Build history of the part. All positions in model axes, mm. A direction names the side the tool comes from. Coordinates: 2 decimals unless noted, no trailing zeros. Write each loop counter-clockwise with the first axis right and the second up, starting at its lowest first coordinate (ties: lowest second). Pieces come first, ordered by that corner, then holes. Notation, with made-up numbers: (-13, -24.75) -> (-2, -24.75) arc R19 cw to (-2, -17.75) -> close; hole circle Ø7 at (87.25, 64.25). An arc over 180 degrees is marked (long way). Write each question's results on one line, items separated by ' | '. Start each with the question number.
Q1. Two-plate mould, pull along Y, no slides. Class faces 1 (the face through (13, 17, 3)), 2 (the face through (10, 24, 6)), 3 (the face through (16.403, 18, 1)), 4 (the face through (11.403, 8, 1)): released by +Y, released by -Y, zero draft, split by the parting line, or undercut.
Q2. Drill centre lines: line 1 (X direction, y = 9.5, z = -2.25); line 2 (Y direction, x = 12, z = 4.5); line 3 (Y direction, x = 4, z = 5.5). Where is each one in solid material? Low to high.
Q3. Tool access for faces 5 (the face through (-11.597, 22, 1)), 6 (the face through (13, 19.5, 3)), 7 (the face through (11.4, 26.22, 1.47)): list every direction of +Z, -Z, +X, -X, +Y, -Y with a clear straight run to the whole face (end or side of a thin tool).
Q4. Saw through at D-D on x = -5.5. Give the cut face in (y, z), and give its area (3 significant figures).
Q5. Saw through at B-B on z = 4.5. Give the cut face in (x, y).
Q6. Saw through at C-C on y = 12. Give the cut face in (x, z).
Q7. Drop flat-ended pins along their axis: pin 1 Ø4 at (x, z) = (13.9, 1.23) entering from -Y; pin 2 Ø0.8 at (y, z) = (4.5, 0) entering from +X; pin 3 Ø2.5 at (x, z) = (-14.1, 1.23) entering from -Y; pin 4 Ø6 at (y, z) = (23, -3) entering from -X. Give the stop position or say it passes through.
Q8. Saw through at A-A on z = 2.25. Count the separate pieces of the cut face and the enclosed holes in it, and give its area (3 significant figures).
from build123d import *

# Parameters (mm, degrees)
SKETCH2_W           = 23
SKETCH2_H           = 12
BOSS_EXTRUDE1_DEPTH = 24
BOSS_EXTRUDE2_DEPTH = 4.5
SKETCH4_R           = 2.5
BOSS_EXTRUDE3_DEPTH = 4
SKETCH5_W           = 12
SKETCH5_H           = 2.5
BOSS_EXTRUDE4_DEPTH = 5
SKETCH6_W           = 12
SKETCH6_H           = 2.5
BOSS_EXTRUDE5_DEPTH = 5
SKETCH7_R           = 1.5
CUT_EXTRUDE1_DEPTH  = 5
SKETCH8_W           = 5.723155949
SKETCH8_H           = 1.635187414
BOSS_EXTRUDE6_DEPTH = 4


with BuildPart() as part:
    # Sketch2 → Boss-Extrude1 (new body)
    with BuildSketch(Plane(origin=(0, 0, 0), x_dir=(1, 0, 0), z_dir=(0, 1, 0))):
        with Locations((-0.097292724, -1.232656514)):
            Rectangle(SKETCH2_W, SKETCH2_H)
    extrude(amount=BOSS_EXTRUDE1_DEPTH)

    # Sketch3 → Boss-Extrude2 (add)
    with BuildSketch(Plane(origin=(0, 24, 0), x_dir=(1, 0, 0), z_dir=(0, 1, 0))):
        with BuildLine():
            ThreePointArc((-0.263959391, -3.204683109), (11.402707276, -1.232656514), (-0.263959391, 0.73937008))
            ThreePointArc((-0.263959391, 0.73937008), (-2.597292724, -1.232656514), (-0.263959391, -3.204683109))
        make_face()
    extrude(amount=BOSS_EXTRUDE2_DEPTH)

    # Sketch4 → Boss-Extrude3 (add)
    with BuildSketch(Plane(origin=(0, 28.5, 0), x_dir=(1, 0, 0), z_dir=(0, 1, 0))):
        with Locations((5.402707276, -1.232656514)):
            Circle(SKETCH4_R)
    extrude(amount=BOSS_EXTRUDE3_DEPTH)

    # Sketch5 → Boss-Extrude4 (add)
    with BuildSketch(Plane(origin=(11.402707276, 0, 0), x_dir=(0, 0, -1), z_dir=(1, 0, 0))):
        with Locations((-1.232656514, 18.25)):
            Rectangle(SKETCH5_W, SKETCH5_H)
    extrude(amount=BOSS_EXTRUDE4_DEPTH)

    # Sketch6 → Boss-Extrude5 (add)
    with BuildSketch(Plane.ZY.offset(11.597292724)):
        with Locations((1.232656514, 18.25)):
            Rectangle(SKETCH6_W, SKETCH6_H)
    extrude(amount=BOSS_EXTRUDE5_DEPTH)

    # Sketch7 → Cut-Extrude1 (cut)
    with BuildSketch(Plane(origin=(0, 19.5, 0), x_dir=(1, 0, 0), z_dir=(0, 1, 0))):
        with Locations((-14.097292724, -1.232656514)):
            Circle(SKETCH7_R)
        with Locations((13.902707276, -1.232656514)):
            Circle(SKETCH7_R)
    extrude(amount=-CUT_EXTRUDE1_DEPTH, mode=Mode.SUBTRACT)

    # Sketch8 → Boss-Extrude6 (add)
    with BuildSketch(Plane(origin=(11.402707276, 0, 0), x_dir=(0, 0, -1), z_dir=(1, 0, 0))):
        with Locations((-1.115857414, 4.321891812)):
            Rectangle(SKETCH8_W, SKETCH8_H)
    extrude(amount=BOSS_EXTRUDE6_DEPTH)


solid = part.part
Returned:
1) face 1: undercut | face 2: released by +Y | face 3: zero draft | face 4: undercut
2) line 1: x = -11.6 to 11.4 | line 2: y = 17 to 19.5 | line 3: y = 0 to 28.5
3) face 5: +Z, -Z, -X, +Y | face 6: +Z, -Z, +X, +Y | face 7: +Y
4) outline: (0, -4.77) -> (24, -4.77) -> (24, 7.23) -> (0, 7.23) -> close | area: 288 mm2
5) outline: (-16.6, 17) -> (-11.6, 17) -> (-11.6, 0) -> (11.4, 0) -> (11.4, 17) -> (16.4, 17) -> (16.4, 19.5) -> (11.4, 19.5) -> (11.4, 24) -> (10.44, 24) -> (10.44, 28.5) -> (0.37, 28.5) -> (0.37, 24) -> (-11.6, 24) -> (-11.6, 19.5) -> (-16.6, 19.5) -> close
6) outline: (-11.6, -4.77) -> (11.4, -4.77) -> (11.4, 7.23) -> (-11.6, 7.23) -> close
7) pin 1: stops at y = 3.5 | pin 2: stops at x = 15.4 | pin 3: passes through | pin 4: stops at x = -11.6
8) separate pieces: 3 | enclosed holes: 0 | area: 652 mm2
